```python
from build123d import *

# Parameters (mm, degrees)
CHAMFER_2_SIZE      = 1
CUT_EXTRUDE_1_DEPTH = 2


with BuildPart() as part:
    # 草图1 → 旋转1 (revolve)
    with BuildSketch(Plane.XY, mode=Mode.PRIVATE) as revolve_1_sk:
        Polygon((0, 0), (3, 0), (3, 8), (2, 8), (2, 10), (4.75, 10), (4.75, 14), (8, 14), (8, 18), (0, 18), align=None)
    revolve(revolve_1_sk.sketch.rotate(Axis((0, 18, 0), (0, -1, 0)), 90), axis=Axis((0, 18, 0), (0, -1, 0)))

    # 倒角2
    chamfer_2_edges = [part.edges().sort_by_distance(p)[0] for p in [
        (0, 8, -3),
        (0, 0, -3),
        (0, 18, -8),
    ]]
    chamfer(chamfer_2_edges, length=CHAMFER_2_SIZE - 0.0001)  # a hair under: the kernel refuses the full size

    # 草图2 → 切除-拉伸1 (cut)
    with BuildSketch(Plane(origin=(0, 18, 0), x_dir=(1, 0, 0), z_dir=(0, 1, 0))):
        with BuildLine():
            Line((-7.964766161, -0.75), (7.964766161, -0.75))
            ThreePointArc((7.964766161, -0.75), (8, 0), (7.964766161, 0.75))
            Line((7.964766161, 0.75), (-7.964766161, 0.75))
            ThreePointArc((-7.964766161, 0.75), (-8, 0), (-7.964766161, -0.75))
        make_face()
    extrude(amount=-CUT_EXTRUDE_1_DEPTH, mode=Mode.SUBTRACT)


solid = part.part
```
Geometry: final body of the model. Coordinates: model frame, mm. A direction names the side the tool comes from. Coordinates: 2 decimals unless noted, no trailing zeros. Order: outer loops, then holes, each group sorted by start corner. A loop starts at its lowest first (then second) coordinate and runs counter-clockwise, first axis right, second up. Notation, with made-up numbers: (62.25, -39.75) -> (109.25, -39.75) arc R25 cw to (109.25, -20.75) -> close; hole circle Ø11 at (-27, 2). An arc over 180 degrees is marked (long way). Answer in a Markdown table with one row per item.
Item 1: Draft query along Z for faces 4 (the conical face through (0.1, 17.8, 7.2)), 5 (the flat face through (0, 16, 0)), 6 (the flat face through (0, 0, 0)), 7 (the cylindrical face through (-0.9, 4.04, 2.86)). Return one class per face: released by +Z, released by -Z, zero draft, split by the parting line, or undercut.
Return value:
| item | result |
|---|---|
| face 4 | released by +Z |
| face 5 | undercut |
| face 6 | zero draft |
| face 7 | split by the parting line |
Item 2: Ray query, L1, parallel to X at y = 15.75, z = -0.25; L2, parallel to Y at x = 4.5, z = -3.25; L3, parallel to Y at x = -3, z = 2. Return the intervals inside material, ascending.
Return value:
| item | result |
|---|---|
| L1 | x = -8 to 8 |
| L2 | y = 14 to 18 |
| L3 | y = 10 to 18 |
Item 3: Access query for faces 1 (the cylindrical face through (2, 9, 0)), 2 (the flat face through (0, 17, -0.75)), 3 (the cylindrical face through (4.637, 12.028, -1.03)). Directions: +Z, -Z, +X, -X, +Y, -Y. A direction counts if a zero-diameter tool reaches every point of the face in a straight line with its end or side. Return the directions, or none.
Return value:
| item | result |
|---|---|
| face 1 | none |
| face 2 | +X, -X, +Y |
| face 3 | -Y |
Item 4: Section C-C on y = 12.75. Output: boundary loops of the cut face in (x, z), plus the area to 3 significant figures.
Return value:
| item | result |
|---|---|
| outline | circle Ø9.5 at (0, 0) |
| area | 70.9 mm² |
Item 5: Section D-D on y = 2. Output: boundary loops of the cut face in (x, z), plus the area to 3 significant figures.
Return value:
| item | result |
|---|---|
| outline | circle Ø6 at (0, 0) |
| area | 28.3 mm² |
Item 6: Contact query for flat-ended pins moving along their axis: P1, Ø3, axis at x = 6.5, y = 14, coming from the +Z side (3 decimals); P2, Ø3, axis at x = -5.5, y = 6, coming from the -Z side; P3, Ø1, axis at x = 1.5, y = 12.5, coming from the -Z side; P4, Ø3, axis at x = 2, y = 6.5, coming from the -Z side. Output: stop coordinate, or through.
Return value:
| item | result |
|---|---|
| P1 | stops at z = 6.245 |
| P2 | passes through |
| P3 | stops at z = -4.64 |
| P4 | stops at z = -2.96 |
